Source: CAD feature listing. Evaluate the final solid. Frame: model axes, mm. Give positions to 0.01 mm unless a question says otherwise; leave off trailing zeros. Loops run counter-clockwise (first coordinate to the right, second up) from the corner with the lowest first, then second, coordinate; pieces in that order, holes last. Notation, with made-up numbers: (61.25, 83) -> (65.25, 83) arc R27 ccw to (65.25, 113) -> close; hole circle Ø10 at (-34.75, 41.5). An arc over 180 degrees is marked (long way). Put each result on its own line as item: value.
```python
from build123d import *

# Parameters (mm, degrees)
BOSS_EXTRUDE1_DEPTH = 1.5
SKETCH2_R           = 8
CUT_EXTRUDE1_DEPTH  = 71.590509277


with BuildPart() as part:
    # Sketch1 → Boss-Extrude1 (new, symmetric)
    with BuildSketch(Plane(origin=(0, 0, 0), x_dir=(0, 0, -1), z_dir=(1, 0, 0))):
        with BuildLine():
            Line((-31, 31.9), (31, 31.9))
            ThreePointArc((31, 31.9), (62.9, 0), (31, -31.9))
            Line((31, -31.9), (-31, -31.9))
            ThreePointArc((-31, -31.9), (-62.9, 0), (-31, 31.9))
        make_face()
    extrude(amount=BOSS_EXTRUDE1_DEPTH, both=True)

    # Sketch2 → Cut-Extrude1 (cut, through all)
    with BuildSketch(Plane(origin=(1.5, 0, 0), x_dir=(0, 0, -1), z_dir=(1, 0, 0))):
        with Locations((-14.3, 0)):
            Circle(SKETCH2_R)
        with Locations((-42.9, 0)):
            Circle(SKETCH2_R)
        with Locations((42.9, 0)):
            Circle(SKETCH2_R)
        with Locations((14.3, 0)):
            Circle(SKETCH2_R)
    extrude(amount=-CUT_EXTRUDE1_DEPTH, mode=Mode.SUBTRACT)


solid = part.part
```
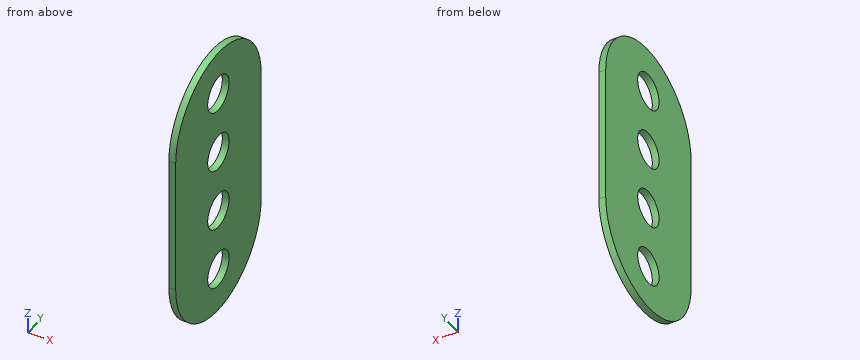
(1) Line query: probe 1 along Y at (x, z) = (-0.15, -14.3); probe 2 along Z at (x, y) = (0.9, 6.5); probe 3 along Z at (x, y) = (0.6, 5) (3 decimals). Output: solid intervals per line, ascending. Write a range as from..to.
Calculated:
probe 1: y = -31.9..-8, 8..31.9
probe 2: z = -62.23..-47.56, -38.24..-18.96, -9.64..9.64, 18.96..38.24, 47.56..62.23
probe 3: z = -62.506..-49.145, -36.655..-20.545, -8.055..8.055, 20.545..36.655, 49.145..62.506
(2) Section A-A on z = 14.3. Return loops of the section in (x, y), then the cut area to 3 significant figures.
Calculated:
outline: (-1.5, -31.9) -> (1.5, -31.9) -> (1.5, -8) -> (-1.5, -8) -> close; (-1.5, 8) -> (1.5, 8) -> (1.5, 31.9) -> (-1.5, 31.9) -> close
area: 143 mm²
(3) Section D-D on y = -18.5. Return loops of the section in (x, z), then the cut area to 3 significant figures.
Calculated:
outline: (-1.5, -56.99) -> (1.5, -56.99) -> (1.5, 56.99) -> (-1.5, 56.99) -> close
area: 342 mm²
(4) First-contact query: P1, Ø14.5, axis at y = 0, z = 14.3, coming from the -X side. Flat tip, straight axial feed; report the tip coordinate or a pass-through.
Calculated:
P1: passes through
(5) Section C-C on z = -42.9. Return loops of the section in (x, y), then the cut area to 3 significant figures.
Calculated:
outline: (-1.5, -29.6) -> (1.5, -29.6) -> (1.5, -8) -> (-1.5, -8) -> close; (-1.5, 8) -> (1.5, 8) -> (1.5, 29.6) -> (-1.5, 29.6) -> close
area: 130 mm²
(6) Section B-B on x = 0. Return loops of the section in (y, z), then the cut area to 3 significant figures.
Calculated:
outline: (-31.9, -31) arc R31.9 ccw to (31.9, -31) -> (31.9, 31) arc R31.9 ccw to (-31.9, 31) -> close; hole circle Ø16 at (0, -42.9); hole circle Ø16 at (0, -14.3); hole circle Ø16 at (0, 14.3); hole circle Ø16 at (0, 42.9)
area: 6,350 mm²
